The drawing under review shows one solid part. Ordinate dimensions are in mm from its lowest x, y, z. A direction names the side the tool comes from. Coordinates: 2 decimals unless noted, no trailing zeros. Write each loop counter-clockwise with the first axis right and the second up, starting at its lowest first coordinate (ties: lowest second). Pieces come first, ordered by that corner, then holes. Notation, with made-up numbers: (68, 5) -> (107, 5) arc R20 ccw to (107, 34) -> close; hole circle Ø11 at (-6, 84.5). An arc over 180 degrees is marked (long way). Put each result on its own line as item: value. Start each with the question number.
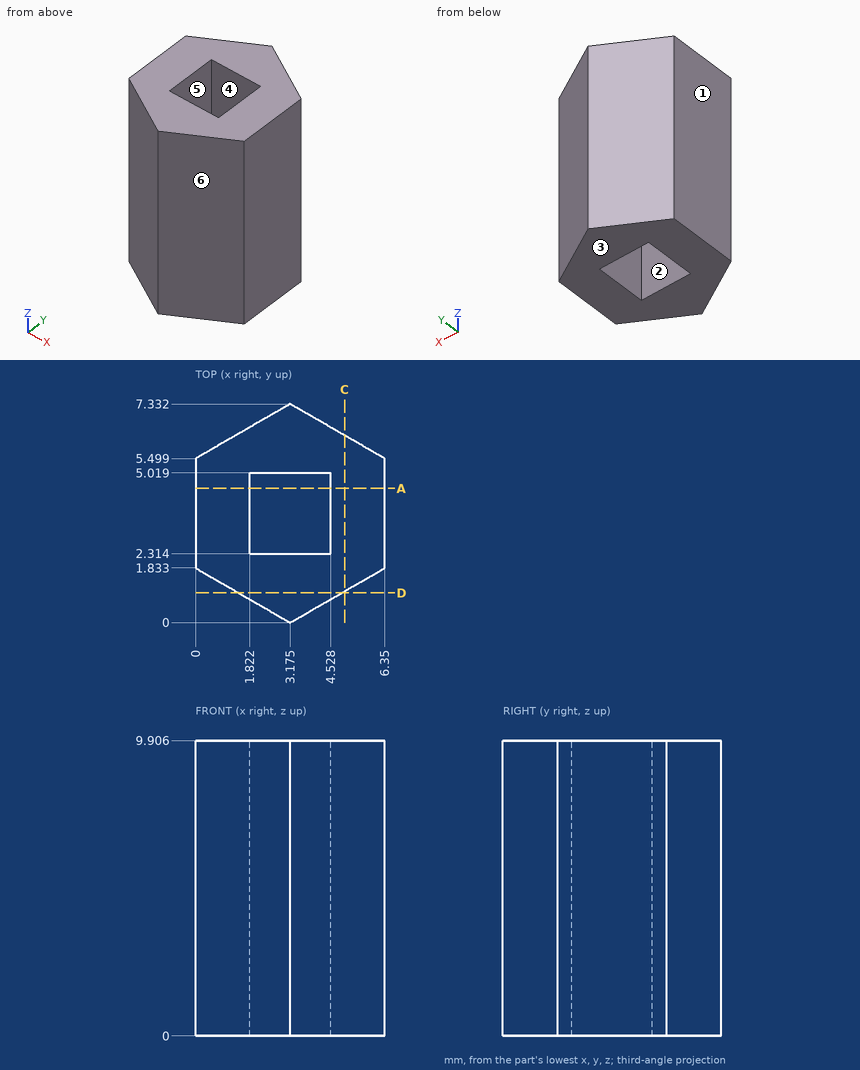
1. The part is to be moulded in two halves that separate along X. For the marked faces 1, 2, 3 and 4, say which applies: released by +X, released by -X, zero draft, split by the parting line, or undercut.
2. Consider section D-D on y = 1. State the section outline as (x, z) points, then the cut area to 3 significant figures.
3. Consider section A-A on y = 4.5. State the section outline as (x, z) points.
4. Tool access review of the marked faces 5 and 6: name each direction out of +Z, -Z, +X, -X, +Y, -Y from which nothing blocks a thin tool from reaching the whole face with its end or side.
5. Wall thickness on line 1 (X direction, y = 3, z = 2); line 2 (Y direction, x = 4, z = 3) (1 decimal); line 3 (Y direction, x = 4.25, z = 3.5) (1 decimal): over which ranges is each line inside the solid? List them lowest first. Write a range as from..to.
6. Insertion check: P1, Ø1, axis at x = 2.5, z = 2, coming from the -Y side; P2, Ø1.5, axis at x = 5.5, z = 4, coming from the +Y side. Each pin has a flat end and moves straight along its axis. Give the tip position at first contact, or say it passes through.
7. Consider section C-C on x = 5. State the section outline as (y, z) points.
Output values:
1. face 1: released by -X
1. face 2: undercut
1. face 3: zero draft
1. face 4: undercut
2. outline: (1.44, 0) -> (4.91, 0) -> (4.91, 9.91) -> (1.44, 9.91) -> close
2. area: 34.3 mm^2
3. outline: (0, 0) -> (1.82, 0) -> (1.82, 9.91) -> (0, 9.91) -> close; (4.53, 0) -> (6.35, 0) -> (6.35, 9.91) -> (4.53, 9.91) -> close
4. face 5: +Z, -Z
4. face 6: +Z, -Z, +X, -Y
5. line 1: x = 0..1.82, 4.53..6.35
5. line 2: y = 0.5..2.3, 5..6.9
5. line 3: y = 0.6..2.3, 5..6.7
6. P1: stops at y = 0.1
6. P2: stops at y = 6.42
7. outline: (1.05, 0) -> (6.28, 0) -> (6.28, 9.91) -> (1.05, 9.91) -> close
